The figure shows three views and two pictorial views of one solid part (mm, origin at its lowest corner). Answer the questions. Coordinates: 2 decimals unless noted, no trailing zeros. Order: outer loops, then holes, each group sorted by start corner. A loop starts at its lowest first (then second) coordinate and runs counter-clockwise, first axis right, second up. Notation, with made-up numbers: M 2.5,60.5 L 43.5,60.5 A27 ccw 43.5,84.5 Z; hole C 22,-4.75 d7. An arc over 180 degrees is marked long. Answer in a Markdown table with one row per item. Add a question column.
Item 1: Consider line 1 (X direction, y = 2.95, z = 53); line 2 (X direction, y = 0.9, z = 28) (1 decimal); line 3 (Z direction, x = 29, y = 3.7) (1 decimal). Determine where each line is inside the solid, lowest interval first. Write a range as from..to.
Item 2: The part is cut by section C-C (y = 2.15). Write down the section's boundary in (x, z).
Item 3: The part is cut by section A-A (x = 13.5). Write down the section's boundary in (y, z).
Item 4: Flat-ended cylindrical pins translate along their axes: pin 1 Ø6.5 at (x, z) = (13.5, 51.68) entering from -Y; pin 2 Ø1 at (x, y) = (107.5, 3) entering from -Z. Find the tip coordinate at first contact, or state that the pin passes through.
Item 5: The part is cut by section D-D (x = 97). Write down the section's boundary in (y, z), then the cut area to 3 significant figures.
Item 6: The part is cut by section B-B (z = 49). Write down the section's boundary in (x, y).
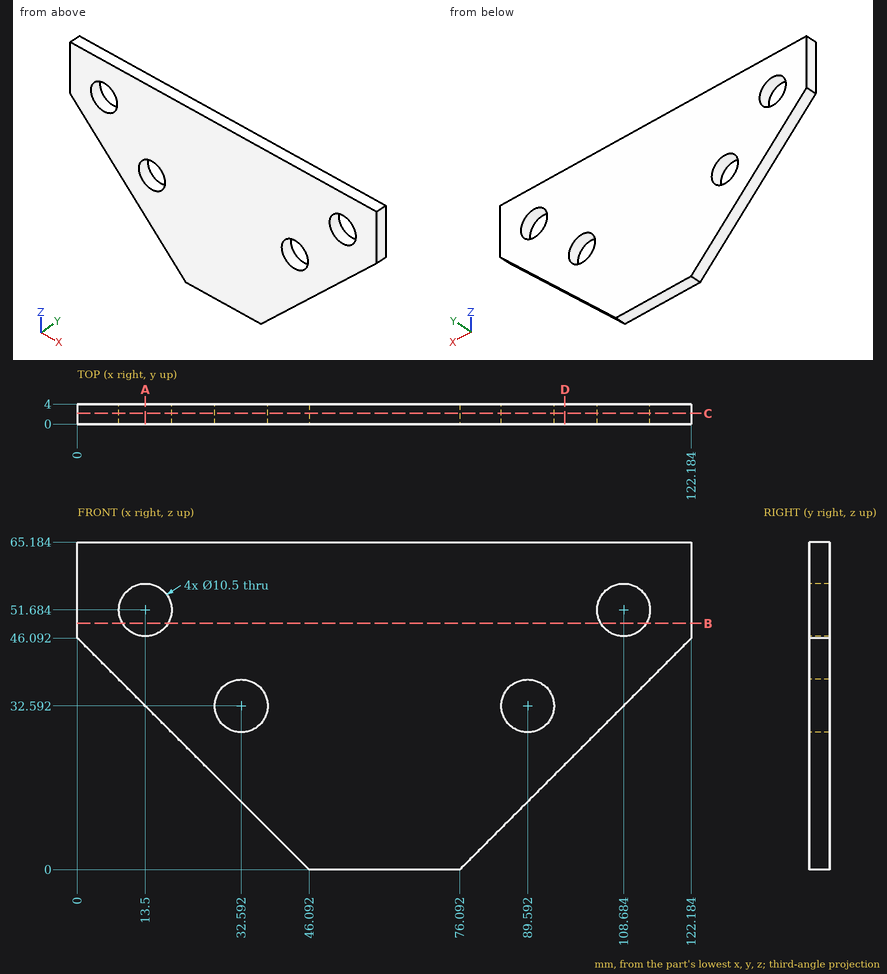
Reply:
| question | item | result |
|---|---|---|
| 1 | line 1 | x = 0..8.42, 18.58..103.6, 113.77..122.18 |
| 1 | line 2 | x = 18.1..30, 35.1..87, 92.1..104.1 |
| 1 | line 3 | z = 17.1..28.8, 36.4..65.2 |
| 2 | outline | M 0,46.09 L 46.09,0 L 76.09,0 L 122.18,46.09 L 122.18,65.18 L 0,65.18 Z; hole C 13.5,51.68 d10.5; hole C 32.59,32.59 d10.5; hole C 89.59,32.59 d10.5; hole C 108.68,51.68 d10.5 |
| 3 | outline | M 0,32.59 L 4,32.59 L 4,46.43 L 0,46.43 Z; M 0,56.93 L 4,56.93 L 4,65.18 L 0,65.18 Z |
| 4 | pin 1 | passes through |
| 4 | pin 2 | stops at z = 30.91 |
| 5 | outline | M 0,20.91 L 4,20.91 L 4,65.18 L 0,65.18 Z |
| 5 | area | 177 mm2 |
| 6 | outline | M 0,0 L 8.99,0 L 8.99,4 L 0,4 Z; M 18.01,0 L 104.17,0 L 104.17,4 L 18.01,4 Z; M 113.2,0 L 122.18,0 L 122.18,4 L 113.2,4 Z |
